Could you check a few things on this model? Use its own coordinates, in mm. Face numbers are marked on the shaded views. A direction names the side the tool comes from. Give positions to 0.01 mm unless a question says otherwise; leave off trailing zeros. Loops run counter-clockwise (first coordinate to the right, second up) from the corner with the lowest first, then second, coordinate; pieces in that order, holes last. Notation, with made-up numbers: (22, -25.75) - (77, -25.75) arc R33 ccw to (77, 3.25) - close; hole circle Ø2 at (51, 73.25). An arc over 180 degrees is marked (long way). Write each question's results on one line, items separated by ' | '. Start each with the question number.
(1) I need wall thicknesses on line 1 (Z direction, x = 5, y = 3); line 2 (Z direction, x = 30, y = 11); line 3 (Z direction, x = -18.5, y = 2.5). Which ranges of each line are inside material? Lowest first, please.
(2) If we mould it in two halves opening along Z, with no side actions, what happens to the marked faces 1, 2 and 3? For each: released by +Z, released by -Z, zero draft, split by the parting line, or undercut.
(3) Suppose I cut it at D-D (z = -4.25). Please give me the cut outline in (x, y).
(4) Suppose I cut it at B-B (z = -9.5). Please give me the cut outline in (x, y).
(5) Suppose I cut it at C-C (x = 21). Please give me the cut outline in (y, z), and give its area (3 significant figures).
(6) For pin 1 (1.5 mm diameter, centred on y = 8, z = -1.5, fed in from +X); pin 2 (4 mm diameter, centred on x = -28.09, z = -9.5, fed in from -Y); pin 3 (0.5 mm diameter, centred on x = -25, y = 10.5, fed in from +Z); pin 4 (1.5 mm diameter, centred on y = 8, z = -10.5, fed in from -X), each with a flat end and sliding along its axis, tell me the tip position at first contact or that it passes through.
(7) On a 3-axis mill with a long thin cutter (end or side, diameter ignored), from which of +Z, -Z, +X, -X, +Y, -Y can I reach the whole of each face in a straight line? I mean the marked faces 4 and 5. Say none if no direction works.
(8) Suppose I cut it at A-A (y = 9). Please give me the cut outline in (x, z).
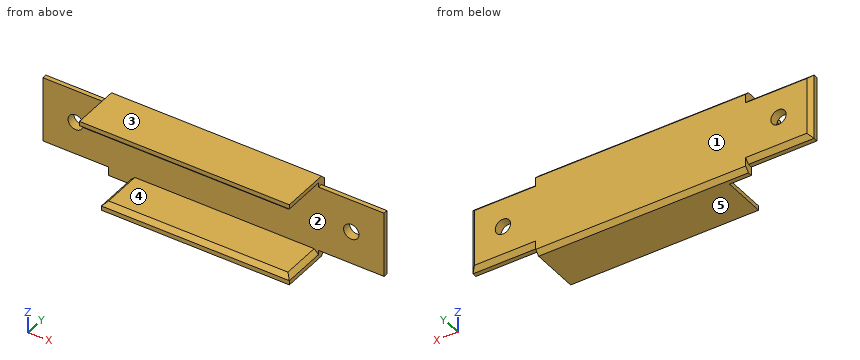
from build123d import *

# Parameters (mm, degrees)
F0_W      = 78
F0_H      = 12
F1_DEPTH  = 19
F2_R      = 1.75
F3_DEPTH  = 10
F3_FACE_W = 15
F3_FACE_H = 2
F2_W      = 15
F2_H      = 2
F4_DEPTH  = 12
F5_SIZE   = 0.99999


# Not quite as in the source:
# - a fillet or chamfer is up to 0.001 mm smaller than in the source, because OpenCascade refuses the exact size


with BuildPart() as f1:
    # F0 (on Top) → F1 (new body)
    with BuildSketch(Plane.XY):
        with Locations((3.4338701516, 6)):
            Rectangle(F0_W, F0_H)
    extrude(amount=-F1_DEPTH)

    # F2 (on face) → F3 (cut)
    with BuildSketch(Plane.XZ):
        Polygon((-35.5661298484, -17), (-20.5661298484, -17), (-20.5661298484, -19), (-15.5661298484, -19), (-15.5661298484, -17), (27.4338701516, -17), (42.4338701516, -17), (42.4338701516, -2), (27.4338701516, -2), (-20.5661298484, -2), (-35.5661298484, -2), align=None)
        with Locations((-28.0890100524, -9.5)):
            Circle(F2_R, mode=Mode.SUBTRACT)
        with Locations((34.9338701516, -9.5)):
            Circle(F2_R, mode=Mode.SUBTRACT)
    extrude(amount=-F3_DEPTH, mode=Mode.SUBTRACT)

    # F3_face (on face) + F2 (on face) → F4 (cut, through all)
    with BuildSketch(Plane(origin=(-28.0661298484, 0, -18), x_dir=(1, 0, 0), z_dir=(0, -1, 0))):
        Rectangle(F3_FACE_W, F3_FACE_H)
    with BuildSketch(Plane.XZ):
        with Locations((-28.0661298484, -1)):
            Rectangle(F2_W, F2_H)
        with Locations((34.9338701516, -1)):
            Rectangle(F2_W, F2_H)
        with Locations((34.9338701516, -18)):
            Rectangle(F2_W, F2_H)
        with Locations((-28.0890100524, -9.5)):
            Circle(F2_R)
        with Locations((34.9338701516, -9.5)):
            Circle(F2_R)
    extrude(amount=-F4_DEPTH, mode=Mode.SUBTRACT)

    # F5 (size 1 in the source; OpenCascade refuses exactly that, so slightly less here)
    f5_edges = [f1.edges().sort_by_distance(p)[0] for p in [
        (-35.56613, 12, -9.5),
        (-28.06613, 12, -2),
        (3.43387, 12, -19),
        (34.93387, 12, -17),
        (42.43387, 12, -9.5),
        (34.93387, 12, -2),
        (3.43387, 12, 0),
        (3.43387, 0, -2),
        (5.93387, 0, -17),
        (27.43387, 5, -17),
        (27.43387, 5, -2),
        (-15.56613, 5, -17),
        (-20.56613, 5, -2),
        (-28.06613, 12, -17),
    ]]
    chamfer(f5_edges, length=F5_SIZE)


solid = f1.part
Output values:
1) line 1: -19 to -17, -2 to 0 | line 2: -17 to -2 | line 3: -2 to 0
2) face 1: zero draft | face 2: undercut | face 3: released by +Z
3) outline: (-35.57, 10) - (42.43, 10) - (42.43, 11) - (41.43, 12) - (-34.57, 12) - (-35.57, 11) - close
4) outline: (-35.57, 10) - (-29.84, 10) - (-29.84, 12) - (-34.57, 12) - (-35.57, 11) - close; (-26.34, 10) - (33.18, 10) - (33.18, 12) - (-26.34, 12) - close; (36.68, 10) - (42.43, 10) - (42.43, 11) - (41.43, 12) - (36.68, 12) - close
5) outline: (0, -19) - (11, -19) - (12, -18) - (12, -1) - (11, 0) - (0, 0) - (0, -1) - (1, -2) - (10, -2) - (10, -17) - (1, -17) - (0, -18) - close | area: 76.0 mm2
6) pin 1: x = 27.43 | pin 2: y = 10 | pin 3: z = -2 | pin 4: through
7) face 4: +X, -X, -Y | face 5: -Z, +X, -X, +Y, -Y
8) outline: (-20.57, -1) - (-19.57, -2) - (26.43, -2) - (27.43, -1) - (27.43, 0) - (-20.57, 0) - close; (-15.57, -19) - (27.43, -19) - (27.43, -18) - (26.43, -17) - (-14.57, -17) - (-15.57, -18) - close
